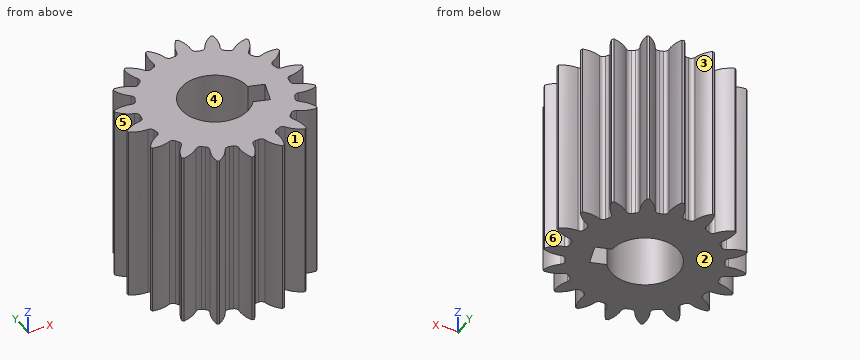
from build123d import *

# Parameters (mm, degrees)
SKETCH3_R         = 20
GEARBODY_DEPTH    = 40
TOOTHCUT_DEPTH    = 49.989794856
CIRPATTERN1_COUNT = 18
BOREDIA_R         = 7.5
BORE_DEPTH        = 12700
KWY1_DEPTH        = 6350


with BuildPart() as part:
    # Sketch3 → gearBody (new body)
    with BuildSketch(Plane.XY):
        Circle(SKETCH3_R)
    extrude(amount=GEARBODY_DEPTH)

    # Sketch2 → toothCut (cut, through all)
    with BuildSketch(Plane.XY):
        with BuildLine():
            ThreePointArc((15.410131867, -2.074959393), (15.458047875, -1.681183079), (15.495903347, -1.286312602))
            ThreePointArc((15.495903347, -1.286312602), (15.763268662, -0.701752182), (16.342213115, -0.422434409))
            ThreePointArc((16.342213115, -0.422434409), (19.177928805, 0.519107216), (21.353959141, 2.566709737))
            ThreePointArc((21.353959141, 2.566709737), (21.381581374, -2.325413473), (20.302931423, -7.097220969))
            ThreePointArc((20.302931423, -7.097220969), (18.617955496, -4.629703952), (16.050944608, -3.100573739))
            ThreePointArc((16.050944608, -3.100573739), (15.545581587, -2.703329086), (15.410131867, -2.074959393))
        make_face()
    toothcut = extrude(amount=TOOTHCUT_DEPTH, mode=Mode.SUBTRACT)

    # CirPattern1: toothCut ×18 about axis
    cirpattern1_axis = Axis((0, 0, 0), (0, 0, 1))
    for i in range(1, CIRPATTERN1_COUNT):
        add(toothcut.rotate(cirpattern1_axis, i * 360 / CIRPATTERN1_COUNT), mode=Mode.SUBTRACT)

    # boreDia → bore (cut, symmetric)
    with BuildSketch(Plane.XY):
        Circle(BOREDIA_R)
    extrude(amount=BORE_DEPTH, both=True, mode=Mode.SUBTRACT)

    # kwy1sketch → kwy1 (cut, symmetric)
    with BuildSketch(Plane.XY):
        Polygon((10.780497106, -0.529983162), (9.384957794, -5.331281948), (3.383334312, -3.586857808), (0, 0), (4.778873624, 1.214440978), align=None)
    extrude(amount=KWY1_DEPTH, both=True, mode=Mode.SUBTRACT)


solid = part.part
Read the model definition and answer for the solid it produces. Units are mm, in the model's axes. Face numbers are marked on the shaded views. A direction names the side the tool comes from. Give positions to 0.01 mm unless a question says otherwise; leave off trailing zeros. Answer as a JSON object with one key per item and string values. Group by question number.
1) Each of these flat-tipped pins is pushed along its axis until it touches: P1, Ø3, axis at y = -9.5, z = 26.5, coming from the -X side; P2, Ø4, axis at x = -14, y = 4.5, coming from the -Z side; P3, Ø1, axis at y = 14, z = 19.5, coming from the +X side; P4, Ø1, axis at x = -12, z = 15, coming from the +Y side. Where does it stop, or does it pass through?
2) Consider L1, parallel to Y at x = 16, z = 7.5; L2, parallel to X at y = -18, z = 34; L3, parallel to Y at x = 0, z = 24. Determine where each line is inside the solid, lowest interval first. Write a range as from..to.
3) A tool of negligible diameter and unlimited length cuts with its end or side. For the marked faces 1, 2 and 3, from which of +Z, -Z, +X, -X, +Y, -Y can it reach the whole face along a straight path? Write none if from no direction.
4) The mould has two halves that part along X. Classify the marked faces 4, 5 and 6: +X half, -X half, draft (parallel to the pull), parting line (faces both ways), or undercut.
Values follow:
{
 "1": {"P1": "stops at x = -18.33", "P2": "stops at z = 0", "P3": "stops at x = 14.61", "P4": "stops at y = 10.99"},
 "2": {"L1": "y = -12..-10.9, -6.14..-3.08, -0.53..2.58, 5.46..8.38", "L2": "x = -8.72..-8.51, -3.11..-0.72, 3.25..5.39", "L3": "y = -15.81..-7.5, 7.5..15.81"},
 "3": {"face 1": "+Z, -Z, -Y", "face 2": "-Z, +X, -X, +Y, -Y", "face 3": "+Z, -Z, +Y"},
 "4": {"face 4": "undercut", "face 5": "-X half", "face 6": "+X half"}
}
